```python
from build123d import *

# Parameters (mm, degrees)
SKETCH_1_R      = 6
SKETCH_1_W      = 17
SKETCH_1_H      = 10
EXTRUDE_1_DEPTH = 13
EXTRUDE_2_DEPTH = 13


with BuildPart() as part:
    # 草图1 → 凸台-拉伸1 (new body)
    with BuildSketch(Plane.XY):
        Polygon((-11, 13), (11, 13), (16, 0), (16, -28), (-16, -28), (-16, 0), align=None)
        with Locations(Location((0, 0, 0), (0, 0, 180))):
            Circle(SKETCH_1_R, mode=Mode.SUBTRACT)
        with Locations((0, -19)):
            Rectangle(SKETCH_1_W, SKETCH_1_H, mode=Mode.SUBTRACT)
    extrude(amount=EXTRUDE_1_DEPTH)

    # 草图2 → 凸台-拉伸2 (add)
    with BuildSketch(Plane.XY.offset(13)):
        Polygon((-8.5, -19), (-16, -19), (-16, -28), (16, -28), (16, -19), (8.5, -19), (8.5, -24), (-8.5, -24), align=None)
    extrude(amount=EXTRUDE_2_DEPTH)


solid = part.part
```
Design review of the part built by this model. Coordinates are the model's own, in mm. A direction names the side the tool comes from. Round coordinates to 2 decimals unless told otherwise and drop trailing zeros. Write each loop counter-clockwise with the first axis right and the second up, starting at its lowest first coordinate (ties: lowest second). Pieces come first, ordered by that corner, then holes. Notation, with made-up numbers: (-40, 72.5) -> (-11, 72.5) arc R23 cw to (-11, 109.5) -> close; hole circle Ø11 at (52.25, -25). An arc over 180 degrees is marked (long way). Answer in a Markdown table with one row per item.
Q1. Take a section at C-C, the plane y = -0.5. State the section outline as (x, z) points.
The answers:
| item | result |
|---|---|
| outline | (-16, 0) -> (-5.98, 0) -> (-5.98, 13) -> (-16, 13) -> close; (5.98, 0) -> (16, 0) -> (16, 13) -> (5.98, 13) -> close |
Q2. Draft analysis for pull direction Y (two halves, no side actions). For faces 1 (the face through (0, -28, 13)), 2 (the face through (12, -19, 19)), 3 (the face through (0, -24, 13)), 4 (the face through (-16, -17, 10)), state which applies: +Y half, -Y half, draft (parallel to the pull), parting line (faces both ways), or undercut.
The answers:
| item | result |
|---|---|
| face 1 | -Y half |
| face 2 | +Y half |
| face 3 | undercut |
| face 4 | draft |
Q3. Take a section at B-B, the plane x = 0. State the section outline as (y, z) points.
The answers:
| item | result |
|---|---|
| outline | (-28, 0) -> (-24, 0) -> (-24, 26) -> (-28, 26) -> close; (-14, 0) -> (-6, 0) -> (-6, 13) -> (-14, 13) -> close; (6, 0) -> (13, 0) -> (13, 13) -> (6, 13) -> close |
Q4. To check wall thickness, follow L1, parallel to Y at x = 0, z = 7; L2, parallel to X at y = -21, z = 21.25; L3, parallel to Y at x = 7, z = 3.5. State the ranges of each line that lie inside material, in increasing order. Write a range as [from, to].
The answers:
| item | result |
|---|---|
| L1 | [-28, -24], [-14, -6], [6, 13] |
| L2 | [-16, -8.5], [8.5, 16] |
| L3 | [-28, -24], [-14, 13] |
Q5. Take a section at D-D, the plane z = 23.75. State the section outline as (x, y) points.
The answers:
| item | result |
|---|---|
| outline | (-16, -28) -> (16, -28) -> (16, -19) -> (8.5, -19) -> (8.5, -24) -> (-8.5, -24) -> (-8.5, -19) -> (-16, -19) -> close |
Q6. Take a section at A-A, the plane z = 8.5. State the section outline as (x, y) points, then the cut area to 3 significant figures.
The answers:
| item | result |
|---|---|
| outline | (-16, -28) -> (16, -28) -> (16, 0) -> (11, 13) -> (-11, 13) -> (-16, 0) -> close; hole (-8.5, -24) -> (8.5, -24) -> (8.5, -14) -> (-8.5, -14) -> close; hole circle Ø12 at (0, 0) |
| area | 964 mm² |
Q7. For faces 5 (the face through (0, -14, 6)), 6 (the face through (-12, -19, 19)), 7 (the face through (13.465, 6.591, 6.409)), list the 3-axis set-ups (+Z, -Z, +X, -X, +Y, -Y) from which the entire face can be reached by the end or side of a thin tool; tool diameter is ignored.
The answers:
| item | result |
|---|---|
| face 5 | +Z, -Z |
| face 6 | +Z, +X, -X, +Y |
| face 7 | +Z, -Z, +X, +Y |
Q8. Clearance check with flat-ended pins moving along their axes: pin 1 Ø12 at (x, y) = (-2.5, -3) entering from +Z; pin 2 Ø2 at (x, z) = (10.5, 19) entering from +Y; pin 3 Ø3 at (y, z) = (4, 13.5) entering from +X; pin 4 Ø7 at (x, y) = (0, 0) entering from +Z. State where each tip first meets the part, or that it passes through.
The answers:
| item | result |
|---|---|
| pin 1 | z = 13 |
| pin 2 | y = -19 |
| pin 3 | x = 15.01 |
| pin 4 | through |
